Geometry: final body of the model. Coordinates: model frame, mm. A direction names the side the tool comes from. Give positions to 0.01 mm unless a question says otherwise; leave off trailing zeros. Write each loop counter-clockwise with the first axis right and the second up, starting at its lowest first coordinate (ties: lowest second). Pieces come first, ordered by that corner, then holes. Notation, with made-up numbers: (57, 54.5) -> (74, 54.5) arc R9 ccw to (74, 64.5) -> close; hole circle Ø7 at (-33, -21). An arc over 180 degrees is marked (long way). Answer in a Markdown table with one row per item. Add a question column.
Item 1: First-contact query: P1, Ø23, axis at y = 19.05, z = -25.4, coming from the -X side; P2, Ø1, axis at x = 44.5, z = -15, coming from the -Y side. Flat tips, straight axial feed; report the tip coordinate or a pass-through.
Item 2: Material intervals for probe 1 along X at (y, z) = (19, -1); probe 2 along Y at (x, z) = (87, -25) (3 decimals); probe 3 along X at (y, z) = (30.5, -45) (3 decimals), sorted ascending. Write a range as from..to.
Item 3: Section query B-B on x = 48. Output: boundary loops of the cut face in (y, z) (3 decimals), plus the area to 3 significant figures.
Item 4: Draft query along Y for faces 1 (the flat face through (44, 19, -47.625)), 2 (the flat face through (34, 41.275, -26)), 3 (the cylindrical face through (76.75, 11.32, -1.61)). Return one class per face: +Y half, -Y half, draft (parallel to the pull), parting line (faces both ways), or undercut.
Item 5: Access query for faces 4 (the cylindrical face through (76.75, 11.32, -49.23)), 5 (the flat face through (3.175, 6, -25)), 6 (the flat face through (55, 40, -35.687)). Directions: +Z, -Z, +X, -X, +Y, -Y. A direction counts if a zero-diameter tool reaches every point of the face in a straight line with its end or side. Return the directions, or none.
Item 6: Section query D-D on y = 19.05. State how many separate pieces and enclosed holes the cut face has, plus the area to 3 significant figures.
Item 7: Section query C-C on y = 33. Output: boundary loops of the cut face in (x, z) (3 decimals), plus the area to 3 significant figures.
Item 8: Section query A-A on z = -25.4. Output: boundary loops of the cut face in (x, y) (3 decimals), plus the area to 3 significant figures.
```python
from build123d import *

# Parameters (mm, degrees)
SKETCH3_W           = 88.9
SKETCH3_H           = 50.8
SKETCH3_W_2         = 82.55
SKETCH3_H_2         = 44.45
BOSS_EXTRUDE2_DEPTH = 38.1
SKETCH4_R           = 12.7
CUT_EXTRUDE1_DEPTH  = 88.9
SKETCH6_W           = 88.9
SKETCH6_H           = 50.8
BOSS_EXTRUDE3_DEPTH = 3.175
SKETCH7_R           = 12.7
CUT_EXTRUDE2_DEPTH  = 50.8
CUT_EXTRUDE3_REACH  = 43.275
SKETCH8_R           = 2.159
SKETCH8_W           = 41.148
SKETCH8_H           = 20.574


with BuildPart() as part:
    # Sketch3 → Boss-Extrude2 (new body)
    with BuildSketch(Plane(origin=(0, 0, 0), x_dir=(1, 0, 0), z_dir=(0, 1, 0))):
        with Locations((44.45, 25.4)):
            Rectangle(SKETCH3_W, SKETCH3_H)
        with Locations((44.45, 25.4)):
            Rectangle(SKETCH3_W_2, SKETCH3_H_2, mode=Mode.SUBTRACT)
    extrude(amount=BOSS_EXTRUDE2_DEPTH)

    # Sketch4 → Cut-Extrude1 (cut)
    with BuildSketch(Plane(origin=(88.9, 0, 0), x_dir=(0, 0, -1), z_dir=(1, 0, 0))):
        with Locations((25.4, 19.05)):
            Circle(SKETCH4_R)
    extrude(amount=-CUT_EXTRUDE1_DEPTH, mode=Mode.SUBTRACT)

    # Sketch6 → Boss-Extrude3 (add)
    with BuildSketch(Plane(origin=(0, 38.1, 0), x_dir=(1, 0, 0), z_dir=(0, 1, 0))):
        with Locations((44.45, 25.4)):
            Rectangle(SKETCH6_W, SKETCH6_H)
    extrude(amount=BOSS_EXTRUDE3_DEPTH)

    # Sketch7 → Cut-Extrude2 (cut)
    with BuildSketch(Plane(origin=(0, 0, -50.8), x_dir=(-1, 0, 0), z_dir=(0, 0, -1))):
        with Locations((-66.675, 19.05)):
            Circle(SKETCH7_R)
        with Locations((-22.225, 19.05)):
            Circle(SKETCH7_R)
    extrude(amount=-CUT_EXTRUDE2_DEPTH, mode=Mode.SUBTRACT)

    # Sketch8 → Cut-Extrude3 (cut, up to next)
    with BuildSketch(Plane(origin=(0, 41.275, 0), x_dir=(1, 0, 0), z_dir=(0, 1, 0)), mode=Mode.PRIVATE) as cut_extrude3_sk1:
        with Locations((31.8135, 31.3055)):
            Circle(SKETCH8_R)
    cut_extrude3_tool1 = extrude(cut_extrude3_sk1.sketch, amount=-CUT_EXTRUDE3_REACH, mode=Mode.PRIVATE) & part.part
    add(cut_extrude3_tool1.solids().sort_by_distance((31.8135, 41.275, -31.3055))[0], mode=Mode.SUBTRACT)
    # Sketch8 → Cut-Extrude3 (cut, up to next)
    with BuildSketch(Plane(origin=(0, 41.275, 0), x_dir=(1, 0, 0), z_dir=(0, 1, 0)), mode=Mode.PRIVATE) as cut_extrude3_sk2:
        with Locations((31.8135, 19.4945)):
            Circle(SKETCH8_R)
    cut_extrude3_tool2 = extrude(cut_extrude3_sk2.sketch, amount=-CUT_EXTRUDE3_REACH, mode=Mode.PRIVATE) & part.part
    add(cut_extrude3_tool2.solids().sort_by_distance((31.8135, 41.275, -19.4945))[0], mode=Mode.SUBTRACT)
    # Sketch8 → Cut-Extrude3 (cut, up to next)
    with BuildSketch(Plane(origin=(0, 41.275, 0), x_dir=(1, 0, 0), z_dir=(0, 1, 0)), mode=Mode.PRIVATE) as cut_extrude3_sk3:
        with Locations((79.4385, 19.4945)):
            Circle(SKETCH8_R)
    cut_extrude3_tool3 = extrude(cut_extrude3_sk3.sketch, amount=-CUT_EXTRUDE3_REACH, mode=Mode.PRIVATE) & part.part
    add(cut_extrude3_tool3.solids().sort_by_distance((79.4385, 41.275, -19.4945))[0], mode=Mode.SUBTRACT)
    # Sketch8 → Cut-Extrude3 (cut, up to next)
    with BuildSketch(Plane(origin=(0, 41.275, 0), x_dir=(1, 0, 0), z_dir=(0, 1, 0)), mode=Mode.PRIVATE) as cut_extrude3_sk4:
        with Locations((79.4385, 31.3055)):
            Circle(SKETCH8_R)
    cut_extrude3_tool4 = extrude(cut_extrude3_sk4.sketch, amount=-CUT_EXTRUDE3_REACH, mode=Mode.PRIVATE) & part.part
    add(cut_extrude3_tool4.solids().sort_by_distance((79.4385, 41.275, -31.3055))[0], mode=Mode.SUBTRACT)
    # Sketch8 → Cut-Extrude3 (cut, up to next)
    with BuildSketch(Plane(origin=(0, 41.275, 0), x_dir=(1, 0, 0), z_dir=(0, 1, 0)), mode=Mode.PRIVATE) as cut_extrude3_sk5:
        with Locations((55.626, 25.4)):
            Rectangle(SKETCH8_W, SKETCH8_H)
    cut_extrude3_tool5 = extrude(cut_extrude3_sk5.sketch, amount=-CUT_EXTRUDE3_REACH, mode=Mode.PRIVATE) & part.part
    add(cut_extrude3_tool5.solids().sort_by_distance((55.626, 41.275, -25.4))[0], mode=Mode.SUBTRACT)


solid = part.part
```
Findings below:
| question | item | result |
|---|---|---|
| 1 | P1 | passes through |
| 1 | P2 | stops at y = 38.1 |
| 2 | probe 1 | x = 0..9.53, 34.92..53.98, 79.37..88.9 |
| 2 | probe 2 | y = 0..6.356, 31.744..41.275 |
| 2 | probe 3 | x = 0..3.175, 85.725..88.9 |
| 3 | outline | (0, -50.8) -> (41.275, -50.8) -> (41.275, -35.687) -> (38.1, -35.687) -> (38.1, -47.625) -> (0, -47.625) -> close; (0, -3.175) -> (38.1, -3.175) -> (38.1, -15.113) -> (41.275, -15.113) -> (41.275, 0) -> (0, 0) -> close |
| 3 | area | 338 mm^2 |
| 4 | face 1 | draft |
| 4 | face 2 | +Y half |
| 4 | face 3 | undercut |
| 5 | face 4 | +Z, -Z |
| 5 | face 5 | -Y |
| 5 | face 6 | +Y, -Y |
| 6 | separate pieces | 6 |
| 6 | enclosed holes | 0 |
| 6 | area | 363 mm^2 |
| 7 | outline | (0, -50.8) -> (88.9, -50.8) -> (88.9, 0) -> (0, 0) -> close; hole (3.175, -47.625) -> (85.725, -47.625) -> (85.725, -3.175) -> (3.175, -3.175) -> close |
| 7 | area | 847 mm^2 |
| 8 | outline | (0, 0) -> (3.175, 0) -> (3.175, 6.35) -> (0, 6.35) -> close; (0, 31.75) -> (3.175, 31.75) -> (3.175, 38.1) -> (35.052, 38.1) -> (35.052, 41.275) -> (0, 41.275) -> close; (76.2, 38.1) -> (85.725, 38.1) -> (85.725, 31.75) -> (88.9, 31.75) -> (88.9, 41.275) -> (76.2, 41.275) -> close; (85.725, 0) -> (88.9, 0) -> (88.9, 6.35) -> (85.725, 6.35) -> close |
| 8 | area | 232 mm^2 |
